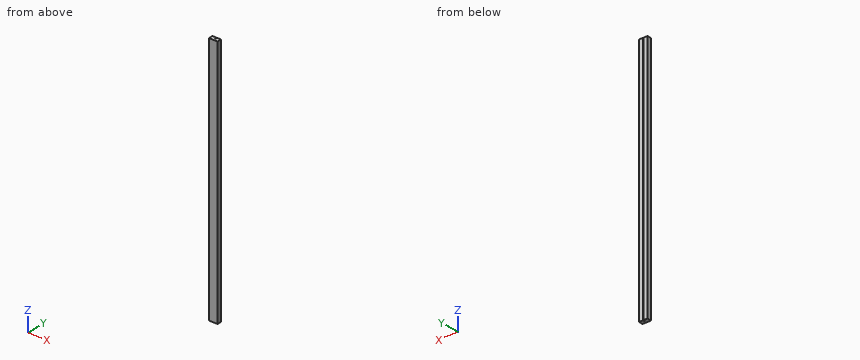
from build123d import *

# Parameters (mm, degrees)
SKETCH1_W           = 101.6
SKETCH1_H           = 50.8
BOSS_EXTRUDE1_DEPTH = 2946.4
CUT_EXTRUDE1_DEPTH  = 19.05


with BuildPart() as part:
    # Sketch1 → Boss-Extrude1 (new body)
    with BuildSketch(Plane.XY):
        with Locations((50.8, 25.4)):
            Rectangle(SKETCH1_W, SKETCH1_H)
    extrude(amount=BOSS_EXTRUDE1_DEPTH)

    # Sketch2 → Cut-Extrude1 (cut)
    with BuildSketch(Plane(origin=(0, 50.8, 0), x_dir=(1, 0, 0), z_dir=(0, 1, 0))):
        Polygon((50.8, -2946.4), (46.0375, -2946.4), (46.0375, 0), (55.5625, 0), (55.5625, -2946.4), align=None)
    extrude(amount=-CUT_EXTRUDE1_DEPTH, mode=Mode.SUBTRACT)


solid = part.part
Build history of the part. All positions in model axes, mm. Coordinates: 2 decimals unless noted, no trailing zeros. Write each loop counter-clockwise with the first axis right and the second up, starting at its lowest first coordinate (ties: lowest second). Pieces come first, ordered by that corner, then holes.
(1) Drill centre line: line 1 (X direction, y = 42, z = 586). Where is it in solid material? Low to high.
(2) Cut at A-A on y = 41. List the corners of the cut face in (x, z), and give its area (3 significant figures).
(3) Cut at B-B on z = 532.5. List the corners of the cut face in (x, y), and give its area (3 significant figures).
Working result:
1. line 1: x = 0 to 46.04, 55.56 to 101.6
2. outline: (0, 0) - (46.04, 0) - (46.04, 2946.4) - (0, 2946.4) - close; (55.56, 0) - (101.6, 0) - (101.6, 2946.4) - (55.56, 2946.4) - close
2. area: 271,000 mm2
3. outline: (0, 0) - (101.6, 0) - (101.6, 50.8) - (55.56, 50.8) - (55.56, 31.75) - (46.04, 31.75) - (46.04, 50.8) - (0, 50.8) - close
3. area: 4,980 mm2
